Autodesk Inventor part; units mm, degrees
ref_plane "YZ Plane" through (0, 0, 0) normal (1, 0, 0) x (0, 1, 0)
ref_plane "XZ Plane" through (0, 0, 0) normal (0, 1, 0) x (-1, 0, 0)
ref_plane "XY Plane" through (0, 0, 0) normal (0, 0, 1) x (1, 0, 0)
sketch "Sketch1" plane through (0, 0, 0) normal (0, 1, 0) x (-1, 0, 0)
  line L0 (0, 0) -> (15.24, 0)
  circle A0 centre (15.24, 0) radius 3.556
  circle A1 centre (0, 0) radius 3.556
  line L1 (18.796, 0) -> (20.066, 0)
  line L2 (15.24, -3.556) -> (15.24, -4.826)
  line L3 (15.24, -4.826) -> (0, -4.826)
  line L4 (-3.556, 0) -> (-4.826, 0)
  line L5 (-4.826, 0) -> (-4.826, -4.826)
  line L6 (-4.826, -4.826) -> (0, -4.826)
  line L7 (15.24, -4.826) -> (20.066, -4.826)
  line L8 (20.066, -4.826) -> (20.066, 0)
  line L9 (15.24, 3.556) -> (15.24, 4.826)
  line L10 (15.24, 4.826) -> (20.066, 4.826)
  line L11 (20.066, 4.826) -> (-4.826, 4.826)
  line L12 (-4.826, 4.826) -> (-4.826, 0)
  line L13 (0, -4.826) -> (-4.826, -4.826)
  line L14 (20.066, 4.826) -> (20.066, 0)
  dimension "d2" = 7.112
  dimension "d0" = 15.24
  dimension "d1" = 7.112
  dimension "d3" = 1.27
  dimension "d4" = 1.27
  dimension "d5" = 1.27
  dimension "d6" = 1.27
extrude "Extrusion1" add sketch "Sketch1" along normal blind 9.652 contours A1 L4 L12 L11 L9 A0 L0 | A1 | L0 A0 L2 L3 L6 L5 L4 A1 | L9 L10 L14 L1 A0 | A0 L1 L8 L7 L2
sketch "Sketch2" plane through (4.826, 0, -4.826) normal (0, 0, -1) x (-1, 0, 0)
  line L0 (0, 0) -> (0, 9.652)
  line L1 (0, 4.826) -> (4.826, 4.826)
  circle A0 centre (4.826, 4.826) radius 3.556
  point P0 (4.826, 0)
  dimension "d9" = 4.826
  dimension "d10" = 7.112
extrude "Extrusion2" cut sketch "Sketch2" against normal through all
sketch "Sketch3" plane through (4.826, 0, 4.826) normal (1, 0, 0) x (0, 0, -1)
  line L0 (4.826, 0) -> (4.826, 9.652)
  line L1 (0, 9.652) -> (9.652, 9.652)
  line L2 (0, 0) -> (0, 9.652)
  line L3 (0, 4.826) -> (9.652, 4.826)
  line L4 (9.652, 0) -> (9.652, 9.652)
  circle A0 centre (4.826, 4.826) radius 5.08
  dimension "d13" = 10.16
extrude "Extrusion3" add sketch "Sketch3" along normal blind 76.2 contours L3 L2 A0 L1 L0 | L3 L4 A0 L2 | L0 L1 A0 L4 L3 | L1 A0 | L2 A0 | L4 A0
sketch "Sketch4" plane through (81.026, 4.826, 0) normal (1, 0, 0) x (0, 0, -1)
  circle A0 centre (0, 0) radius 5.08
  point P0 (0, -4.826)
extrude "Extrusion4" cut sketch "Sketch4" against normal blind 76.2
properties part number "newblockwithnopeg"
Part model, mm, in its own coordinate system. Coordinates: 2 decimals unless noted, no trailing zeros. Order: outer loops, then holes, each group sorted by start corner. A loop starts at its lowest first (then second) coordinate and runs counter-clockwise, first axis right, second up. Notation, with made-up numbers: (-20, -21.75) - (15, -21.75) arc R14 ccw to (15, -10.75) - close; hole circle Ø11 at (10, 22). An arc over 180 degrees is marked (long way). Return JSON: item names as keys, results as strings. Group by question number.
Item 1: Drill centre lines: probe 1 along X at (y, z) = (4.75, 0); probe 2 along X at (y, z) = (7.5, -2); probe 3 along Y at (x, z) = (0, -2.75). Where is each one in solid material? Low to high. Write a range as from..to.
Item 2: Cut at A-A (z = 0). List the corners of the cut face in (x, y).
Item 3: Pull direction X, two halves, no side cores. Call faces 1 (the face through (-20.066, 5, 0)), 2 (the face through (-11, 5, 4.826)), 3 (the face through (0.771, 1.355, -0.068)): pulls with the +X half, pulls with the -X half, needs draft (parallel to the pull), parting line crosses it, or undercut.
Item 4: Cut at D-D (y = 8.75). List the corners of the cut face in (x, z).
Item 5: Cut at B-B (x = 0). List the corners of the cut face in (y, z), plus the area to 3 significant figures.
Item 6: Cut at C-C (y = 5.5). List the corners of the cut face in (x, z), plus the area to 3 significant figures.
Check values:
{
 "1": {"probe 1": "x = -20.07..-18.8, -11.68..-3.56, 3.56..4.83", "probe 2": "x = -20.07..-18.18, -12.3..-2.34, 2.34..4.83", "probe 3": "y = 0..1.27, 8.38..9.65"},
 "2": {"outline": "(-20.07, 0) - (-18.8, 0) - (-18.8, 9.65) - (-20.07, 9.65) - close; (-11.68, 0) - (4.83, 0) - (4.83, 9.65) - (-11.68, 9.65) - close; hole circle Ø7.11 at (0, 4.83)"},
 "3": {"face 1": "pulls with the -X half", "face 2": "needs draft", "face 3": "undercut"},
 "4": {"outline": "(-20.07, -4.83) - (4.83, -4.83) - (4.83, 4.83) - (-20.07, 4.83) - close; hole circle Ø7.11 at (-15.24, 0)"},
 "5": {"outline": "(0, -4.83) - (1.27, -4.83) - (1.27, 4.83) - (0, 4.83) - close; (8.38, -4.83) - (9.65, -4.83) - (9.65, 4.83) - (8.38, 4.83) - close", "area": "24.5 mm2"},
 "6": {"outline": "(-20.07, -4.83) - (-3.49, -4.83) - (-3.49, 4.83) - (-20.07, 4.83) - close; (3.49, -4.83) - (4.83, -4.83) - (4.83, 4.83) - (3.49, 4.83) - close; hole circle Ø7.11 at (-15.24, 0)", "area": "133 mm2"}
}
